For this review, take the finished solid that the model builds, in its own axes (mm). A direction names the side the tool comes from. Give positions to 0.01 mm unless a question says otherwise; leave off trailing zeros. Write each loop counter-clockwise with the first axis right and the second up, starting at its lowest first coordinate (ties: lowest second). Pieces come first, ordered by that corner, then holes.
1) Draft analysis for pull direction Z (two halves, no side actions). For faces 4 (the face through (-20, 0, 141.98)), 5 (the face through (0, 0, 134)), 6 (the face through (-10, 0, 114.86)), state which applies: pulls with the +Z half, pulls with the -Z half, needs draft (parallel to the pull), parting line crosses it, or undercut.
2) Wall thickness on line 1 along Z through (x, y) = (-13, 5.5); line 2 along Y through (x, z) = (-3, 91); line 3 along Z through (x, y) = (-2.5, 1.5): over which ranges is each line inside the solid? List them lowest first.
3) We need section A-A on x = -18. Give the boundary of the cut face in (y, z).
4) For P1, Ø4.5, axis at y = -4.5, z = 23, coming from the +X side; P2, Ø3, axis at y = -2, z = 90, coming from the +X side; P3, Ø3, axis at y = 3, z = 48.5, coming from the +X side, all flat-tipped, find the tip position at first contact; note any pin that passes through.
5) We need section B-B on y = 7.25. Give the boundary of the cut face in (x, z), and give its area (3 significant figures).
6) Machinability: for faces 1 (the face through (-10, 0, 17.11)), 2 (the face through (-40, 0, 72)), 3 (the face through (-5, 1, 53)), which of the approach directions +Z, -Z, +X, -X, +Y, -Y give a long, thin tool a straight path to every point of the face, cutting with its end or side? Answer none if there is none.
from build123d import *

# Parameters (mm, degrees)
F1_DEPTH = 40
F3_DEPTH = 5
F4_DEPTH = 40.001
F6_W     = 20
F6_H     = 10
F7_DEPTH = 25
F8_SIZE  = 0.3


with BuildPart() as f1:
    # F0 (on Right) → F1 (new body)
    with BuildSketch(Plane.YZ):
        Polygon((-10, 0), (0, 0), (10, 0), (10, 141.98), (-10, 141.98), align=None)
    extrude(amount=-F1_DEPTH)

    # F2 (on Right) → F3 (cut)
    with BuildSketch(Plane.YZ):
        with BuildLine():
            ThreePointArc((5, 91.49), (-3.5355339059, 95.0255339059), (0, 86.49))
            ThreePointArc((0, 86.49), (3.5355339059, 87.9544660941), (5, 91.49))
        make_face()
        with BuildLine():
            ThreePointArc((2.5, 91.49), (1.767766953, 89.722233047), (0, 88.99))
            ThreePointArc((0, 88.99), (-1.767766953, 93.257766953), (2.5, 91.49))
        make_face(mode=Mode.SUBTRACT)
        with BuildLine():
            Line((0, 47.99), (0, 45.49))
            ThreePointArc((0, 45.49), (3.5355339059, 46.9544660941), (5, 50.49))
            ThreePointArc((5, 50.49), (3.5355339059, 54.0255339059), (0, 55.49))
            Line((0, 55.49), (0, 52.99))
            ThreePointArc((0, 52.99), (1.767766953, 52.257766953), (2.5, 50.49))
            ThreePointArc((2.5, 50.49), (1.767766953, 48.722233047), (0, 47.99))
        make_face()
        with BuildLine():
            ThreePointArc((0, 55.49), (-5, 50.49), (0, 45.49))
            Line((0, 45.49), (0, 47.99))
            ThreePointArc((0, 47.99), (-2.5, 50.49), (0, 52.99))
            Line((0, 52.99), (0, 55.49))
        make_face()
    extrude(amount=-F3_DEPTH, mode=Mode.SUBTRACT)

    # F4 (cut, through all): faces of the model
    f4_faces = [f1.faces().sort_by_distance(p)[0] for p in [
        (0, 0, 91.49),
        (0, 0, 50.49),
    ]]
    extrude(f4_faces, amount=-F4_DEPTH, mode=Mode.SUBTRACT)

    # F6 (on offset) → F7 (cut)
    with BuildSketch(Plane.XZ.offset(10)):
        with Locations((-10, 119.86)):
            Rectangle(F6_W, F6_H)
        with Locations((-10, 22.11)):
            Rectangle(F6_W, F6_H)
    extrude(amount=-F7_DEPTH, mode=Mode.SUBTRACT)

    # F8
    f8_edges = [f1.edges().sort_by_distance(p)[0] for p in [
        (0, 0, 0),
        (0, -10, 8.555),
        (0, 0, 17.11),
        (0, 10, 8.555),
        (0, 0, 27.11),
        (0, -10, 70.985),
        (0, 0, 114.86),
        (0, 10, 70.985),
        (0, 0, 45.49),
        (0, -5, 91.49),
        (0, 0, 124.86),
        (0, -10, 133.42),
        (0, 0, 141.98),
        (0, 10, 133.42),
        (-20, -10, 0),
        (-40, 0, 0),
        (-20, 10, 0),
        (-20, 10, 141.98),
        (-20, -10, 141.98),
        (-40, 0, 141.98),
        (-10, -10, 124.86),
        (-20, 0, 124.86),
        (-10, 10, 124.86),
        (-20, 0, 114.86),
        (-10, -10, 114.86),
        (-10, 10, 114.86),
        (-10, -10, 27.11),
        (-20, 0, 27.11),
        (-10, 10, 27.11),
        (-10, -10, 17.11),
        (-10, 10, 17.11),
        (-20, 0, 17.11),
        (-20, -10, 119.86),
        (-20, -10, 22.11),
        (-20, 10, 22.11),
        (-20, 10, 119.86),
    ]]
    chamfer(f8_edges, length=F8_SIZE)


solid = f1.part
Results list:
1. face 4: pulls with the +Z half
1. face 5: needs draft
1. face 6: undercut
2. line 1: z = 0 to 17.11, 27.11 to 114.86, 124.86 to 141.98
2. line 2: y = -10 to -4.98, 4.98 to 10
2. line 3: z = 0 to 17.11, 27.11 to 45.72, 55.26 to 86.72, 96.26 to 114.86, 124.86 to 141.98
3. outline: (-10, 0.3) - (-9.7, 0) - (9.7, 0) - (10, 0.3) - (10, 16.81) - (9.7, 17.11) - (-9.7, 17.11) - (-10, 16.81) - close; (-10, 27.41) - (-9.7, 27.11) - (9.7, 27.11) - (10, 27.41) - (10, 114.56) - (9.7, 114.86) - (-9.7, 114.86) - (-10, 114.56) - close; (-10, 125.16) - (-9.7, 124.86) - (9.7, 124.86) - (10, 125.16) - (10, 141.68) - (9.7, 141.98) - (-9.7, 141.98) - (-10, 141.68) - close; hole circle Ø5 at (0, 50.49); hole circle Ø5 at (0, 91.49)
4. P1: stops at x = -20
4. P2: stops at x = -5
4. P3: stops at x = -0.2
5. outline: (-40, 0.3) - (-39.7, 0) - (-0.3, 0) - (0, 0.3) - (0, 16.81) - (-0.3, 17.11) - (-19.7, 17.11) - (-20, 17.41) - (-20, 26.81) - (-19.7, 27.11) - (-0.3, 27.11) - (0, 27.41) - (0, 114.56) - (-0.3, 114.86) - (-19.7, 114.86) - (-20, 115.16) - (-20, 124.56) - (-19.7, 124.86) - (-0.3, 124.86) - (0, 125.16) - (0, 141.68) - (-0.3, 141.98) - (-39.7, 141.98) - (-40, 141.68) - close
5. area: 5,280 mm2
6. face 1: +X, +Y, -Y
6. face 2: +Z, -Z, -X, +Y, -Y
6. face 3: +X
